The model under review builds one solid part; all positions refer to its coordinate system, in mm. A direction names the side the tool comes from. Coordinates: 2 decimals unless noted, no trailing zeros. Order: outer loops, then holes, each group sorted by start corner. A loop starts at its lowest first (then second) coordinate and runs counter-clockwise, first axis right, second up. Notation, with made-up numbers: (8, 21.5) - (22, 21.5) arc R17 ccw to (22, 31.5) - close; hole circle Ø6 at (-12.75, 46.5). An arc over 180 degrees is marked (long way). Answer in a Markdown table with one row per item.
Autodesk Inventor part; units mm, degrees
ref_plane "Work Plane1" through (0, 6.5786, -9.6139) normal (0, 0, 1) x (1, 0, 0)
ref_plane "Work Plane3" through (25.7556, -6.5786, -19.2278) normal (1, 0, 0) x (0, 0, -1)
ref_plane "YZ Plane" through (0, 0, 0) normal (1, 0, 0) x (0, 1, 0)
sketch "Sketch1" plane through (0, 0, 0) normal (0, 1, 0) x (-1, 0, 0)
  line L0 (0, 0) -> (-17.5768, 0)
  line L1 (-17.5768, 0) -> (-17.5768, -19.2278)
  line L2 (-17.5768, -19.2278) -> (0, -19.2278)
  line L3 (0, -19.2278) -> (0, 0)
  dimension "d0" = 17.5768
  dimension "d1" = 19.2278
extrude "Extrusion1" add sketch "Sketch1" along normal mid plane 13.1572
sketch "Sketch4" plane through (0, -6.5786, 0) normal (0, -1, 0) x (1, 0, 0)
  line L0 (17.5768, 0) -> (17.5768, -19.2278)
  circle A0 centre (9.4742, -9.6139) radius 5.3213
  point P0 (0, 0)
  dimension "d12" = 10.6426
extrude "Extrusion4" add sketch "Sketch4" along normal blind 10.2616
sketch "Sketch5" plane through (9.4742, -16.8402, -9.6139) normal (0, -1, 0) x (1, 0, 0)
  circle A0 centre (0, 0) radius 6.1595
  point P0 (-9.4742, 9.6139)
  dimension "d15" = 12.319
extrude "Extrusion5" add sketch "Sketch5" along normal blind 0.8382
sketch "Sketch2" plane through (0, 6.5786, 0) normal (0, 1, 0) x (1, 0, 0)
  line L0 (0, 19.2278) -> (0, 0)
  line L1 (17.5768, 19.2278) -> (0, 19.2278)
  line L2 (0, 0) -> (17.5768, 0)
  line L3 (17.5768, 0) -> (17.5768, 19.2278)
  line L4 (17.5768, 0) -> (9.4742, 0)
  circle A0 centre (9.4742, 9.6139) radius 5.3213
  dimension "d4" = 8.1026
  dimension "d5" = 10.6426
extrude "Extrusion2" add sketch "Sketch2" along normal blind 7.0612 contours A0
sketch "Sketch3" plane through (9.4742, 13.6398, -9.6139) normal (0, 1, 0) x (1, 0, 0)
  circle A0 centre (0, 0) radius 5.8674
  point P0 (-9.4742, -9.6139)
  dimension "d8" = 11.7348
extrude "Extrusion3" add sketch "Sketch3" against normal blind 3.2512
sketch "Sketch7" plane through (0, -6.5786, 0) normal (-1, 0, 0) x (0, 0, 1)
  line L0 (-19.2278, 13.1572) -> (0, 0) construction
  line L1 (-19.2278, 0) -> (-19.2278, 13.1572)
  line L2 (-19.2278, 6.5786) -> (-9.6139, 6.5786) construction
  circle A0 centre (-9.6139, 6.5786) radius 5.715
  point P0 (0, 6.5786)
  dimension "d21" = 11.43
extrude "Extrusion7" add sketch "Sketch7" along normal blind 2.286
sketch "Sketch8" plane through (-2.286, 0, -9.6139) normal (-1, 0, 0) x (0, 0, 1)
  circle A0 centre (0, 0) radius 6.9596
  point P0 (9.6139, 0)
  dimension "d24" = 13.9192
extrude "Extrusion8" add sketch "Sketch8" against normal blind 0.6858
sketch "Sketch6" plane through (9.4742, -17.6784, -9.6139) normal (0, -1, 0) x (1, 0, 0)
  circle A0 centre (0, 0) radius 4.953
  point P0 (-9.4742, 9.6139)
  dimension "d18" = 9.906
extrude "Extrusion6" add sketch "Sketch6" along normal blind 8.763
sketch "Sketch9" plane through (0, 0, 0) normal (0, 0, 1) x (1, 0, 0)
  point P0 (0, 0)
ref_plane "Work Plane1" through (0, 6.5786, -9.6139) normal (0, 0, 1) x (1, 0, 0)
sketch "Sketch11" plane through (0, 0, 0) normal (0, 1, 0) x (-1, 0, 0)
  line L0 (-25.7556, -5.4737) -> (-25.7556, -13.7541)
  line L1 (-25.7556, -9.6139) -> (-21.4884, -9.6139)
  circle A0 centre (-21.4884, -9.6139) radius 2.2225
  point P0 (0, 0)
  dimension "d31" = 4.2672
  dimension "d32" = 4.445
extrude "Extrusion9" add sketch "Sketch11" along normal blind 9.525
ref_plane "Work Plane3" through (25.7556, -6.5786, -19.2278) normal (1, 0, 0) x (0, 0, -1)
sketch "Sketch12" plane through (17.5768, -6.5786, -19.2278) normal (1, 0, 0) x (0, 0, -1)
  point P0 (-19.2278, 6.5786)
sketch "Sketch13" plane through (17.5768, -6.5786, -19.2278) normal (1, 0, 0) x (0, 0, -1)
  circle A0 centre (-9.7674, 6.5786) radius 6.4008
  point P0 (-19.2278, 6.5786)
  dimension "d36" = 12.8016
sketch "Sketch14" plane through (25.7556, -6.5786, -19.2278) normal (1, 0, 0) x (0, 0, -1)
  line L0 (-11.8364, 6.5786) -> (-7.3914, 6.5786)
  circle A0 centre (-9.6139, 6.5786) radius 4.1402
  point P0 (-19.2278, 6.5786)
  dimension "d37" = 8.2804
loft "Loft1" add profiles "Sketch13", "Sketch14"
chamfer "Chamfer1" distance 3.175 angle 45 4 edges at (8.7884, 6.5786, -19.2278) (8.7884, -6.5786, -19.2278) (8.7884, -6.5786, 0) (8.7884, 6.5786, 0)
hole "Hole1" at (-2.286, 0, -9.6139) direction (1, 0, 0) diameter 10.5918 depth 16.8402
hole "Hole2" at (9.4742, 13.6398, -9.6139) direction (0, -1, 0) diameter 9.0678 end through all
hole "Hole3" at (25.7556, 0, -9.6139) direction (-1, 0, 0) diameter 6.8072 end through all
hole "Hole4" at (21.4884, 9.525, -9.6139) direction (0, -1, 0) diameter 3.302 depth 10.16 tip angle 118
properties part number "Carburetor Housing" material "Lead"
Item 1: Clearance check with flat-ended pins moving along their axes: pin 1 Ø3 at (x, y) = (5, -9) entering from +Z; pin 2 Ø9 at (y, z) = (0, -9.61) entering from +X; pin 3 Ø8.5 at (y, z) = (0, -9.61) entering from -X; pin 4 Ø4 at (y, z) = (-9, -12) entering from +X. State where each tip first meets the part, or that it passes through.
Check values:
| item | result |
|---|---|
| pin 1 | z = -5.2 |
| pin 2 | x = 25.76 |
| pin 3 | x = 14.55 |
| pin 4 | x = 14.78 |
Item 2: We need section B-B, the plane y = -16. Write out the cut boundary in (x, z).
Check values:
| item | result |
|---|---|
| outline | circle Ø10.64 at (9.47, -9.61); hole circle Ø9.07 at (9.47, -9.61) |
Item 3: To check wall thickness, follow line 1 (Z direction, x = 1.5, y = 0); line 2 (Y direction, x = 15, z = -7.25); line 3 (Y direction, x = 4.75, z = -9.5). State the ranges of each line that lie inside material, in increasing order. Write a range as from..to.
Check values:
| item | result |
|---|---|
| line 1 | -19.23..-14.91, -4.32..0 |
| line 2 | -17.68..-16.84, -6.58..-2.45, 2.45..6.58 |
| line 3 | -26.44..-5.29, 5.29..13.64 |
Item 4: We need section C-C, the plane z = -1.5. Write out the cut boundary in (x, y), then the cut area to 3 significant figures.
Check values:
| item | result |
|---|---|
| outline | (0, -4.9) - (17.58, -4.9) - (17.58, 4.9) - (0, 4.9) - close |
| area | 172 mm^2 |
Item 5: Mouldability with a two-part tool opening along X and no side actions: class faces 6 (the face through (5, -6.579, -5)), 7 (the face through (4, -16.84, -11)), 8 (the face through (14.894, 12.037, -7.367)) as +X half, -X half, draft (parallel to the pull), parting line (faces both ways), or undercut.
Check values:
| item | result |
|---|---|
| face 6 | undercut |
| face 7 | draft |
| face 8 | parting line |
Item 6: We need section A-A, the plane z = -10.5. State how many separate pieces and enclosed holes the cut face has, then the cut area to 3 significant figures.
Check values:
| item | result |
|---|---|
| separate pieces | 5 |
| enclosed holes | 0 |
| area | 112 mm^2 |
Item 7: Tool access review of faces 1 (the face through (-0.79, -3.86, -13.83)), 2 (the face through (25.756, -3, -7)), 3 (the face through (-1.948, 2.09, -2.976)), 4 (the face through (5, -17.678, -7)), 5 (the face through (8.67, -5.01, -17.62)): name each direction out of +Z, -Z, +X, -X, +Y, -Y from which nothing blocks a thin tool from reaching the whole face with its end or side.
Check values:
| item | result |
|---|---|
| face 1 | none |
| face 2 | +Z, -Z, +X, +Y, -Y |
| face 3 | -X |
| face 4 | -Y |
| face 5 | -Z, +X, -X, -Y |
